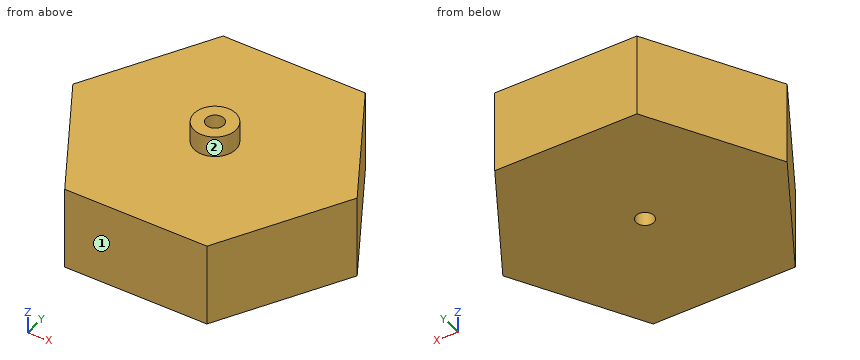
```python
from build123d import *

# Parameters (mm, degrees)
BOSS_EXTRUDE1_DEPTH = 4
SKETCH2_R           = 1
SKETCH2_R_2         = 0.425
BOSS_EXTRUDE2_DEPTH = 1
SKETCH6_R           = 0.425
CUT_EXTRUDE1_DEPTH  = 63


with BuildPart() as part:
    # Sketch1 → Boss-Extrude1 (new body)
    with BuildSketch(Plane.XY):
        Polygon((3.4, 0), (-3.4, 0), (-6.8, -5.888972746), (-3.4, -11.777945491), (3.4, -11.777945491), (6.8, -5.888972746), align=None)
    extrude(amount=BOSS_EXTRUDE1_DEPTH)

    # Sketch2 → Boss-Extrude2 (add)
    with BuildSketch(Plane.XY.offset(4)):
        with Locations((0, -5.888972746)):
            Circle(SKETCH2_R)
        with Locations((0, -5.888972746)):
            Circle(SKETCH2_R_2, mode=Mode.SUBTRACT)
    extrude(amount=BOSS_EXTRUDE2_DEPTH)

    # Sketch6 → Cut-Extrude1 (cut)
    with BuildSketch(Plane.XY.offset(4)):
        with Locations((0, -5.888972746)):
            Circle(SKETCH6_R)
    extrude(amount=-CUT_EXTRUDE1_DEPTH, mode=Mode.SUBTRACT)


solid = part.part
```
Build history of the part. All positions in model axes, mm. Face numbers are marked on the shaded views. A direction names the side the tool comes from. Give positions to 0.01 mm unless a question says otherwise; leave off trailing zeros. Loops run counter-clockwise (first coordinate to the right, second up) from the corner with the lowest first, then second, coordinate; pieces in that order, holes last. Notation, with made-up numbers: (60.5, 87) -> (105.5, 87) arc R18 cw to (105.5, 122) -> close; hole circle Ø8 at (54.5, 89.25). An arc over 180 degrees is marked (long way). One line per question, with ' | ' between items. Start each with the question number.
1) 3-axis set-ups, long thin cutter, end or side, ignore diameter. For the marked faces 1 and 2: which of +Z, -Z, +X, -X, +Y, -Y reach the whole face in a straight line?
2) Cut at C-C (x = 1.5). Give the cut face in (y, z).
3) Cut at B-B (z = 0.9). Give the cut face in (x, y) (3 decimals).
4) Cut at D-D (y = -2.5). Give the cut face in (x, z), plus the area to 3 significant figures.
5) Cut at A-A (x = 0). Give the cut face in (y, z).
6) Pin check, flat tips, straight feed: pin 1 (1.5 mm diameter, centred on y = -7, z = 3.5, fed in from -X); pin 2 (1.5 mm diameter, centred on x = -4.5, y = -3, fed in from +Z); pin 3 (1.5 mm diameter, centred on x = 4.5, z = 1.5, fed in from -Y). Stop position of each tip, or through.
7) Probe L1, parallel to Y at x = 0, z = 4.6; L2, parallel to Y at x = 0, z = 2.8; L3, parallel to Z at x = 4.5, y = -3.75. List the from-to ranges inside material, lowest first.
Return value:
1) face 1: +Z, -Z, +X, -X, -Y | face 2: +Z
2) outline: (-11.78, 0) -> (0, 0) -> (0, 4) -> (-11.78, 4) -> close
3) outline: (-6.8, -5.889) -> (-3.4, -11.778) -> (3.4, -11.778) -> (6.8, -5.889) -> (3.4, 0) -> (-3.4, 0) -> close; hole circle Ø0.85 at (0, -5.889)
4) outline: (-4.84, 0) -> (4.84, 0) -> (4.84, 4) -> (-4.84, 4) -> close | area: 38.7 mm^2
5) outline: (-11.78, 0) -> (-6.31, 0) -> (-6.31, 5) -> (-6.89, 5) -> (-6.89, 4) -> (-11.78, 4) -> close; (-5.46, 0) -> (0, 0) -> (0, 4) -> (-4.89, 4) -> (-4.89, 5) -> (-5.46, 5) -> close
6) pin 1: x = -6.59 | pin 2: z = 4 | pin 3: y = -11.17
7) L1: -6.89 to -6.31, -5.46 to -4.89 | L2: -11.78 to -6.31, -5.46 to 0 | L3: 0 to 4
